```python
from build123d import *

# Parameters (mm, degrees)
EXTRUDE_1_DEPTH         = 13
HOLE_WIZARD_6_2_6_2_1_D = 6.2
HOLE_WIZARD_6_2_6_2_2_D = 6.2
FILLET_1_R              = 3


with BuildPart() as part:
    # 草图1 → 凸台-拉伸1 (new, symmetric)
    with BuildSketch(Plane.XY):
        Polygon((0, 0), (30, 0), (30, 4), (4, 4), (4, 30), (0, 30), align=None)
    extrude(amount=EXTRUDE_1_DEPTH, both=True)

    # Ø6.2 (6.2) 直径孔1 (through all)
    with Locations(Plane(origin=(0, 4, 0), x_dir=(1, 0, 0), z_dir=(0, 1, 0))):
        with Locations((15, 0)):
            Hole(HOLE_WIZARD_6_2_6_2_1_D / 2)

    # Ø6.2 (6.2) 直径孔2 (through all)
    with Locations(Plane(origin=(4, 0, 0), x_dir=(0, 0, -1), z_dir=(1, 0, 0))):
        with Locations((0, 15)):
            Hole(HOLE_WIZARD_6_2_6_2_2_D / 2)

    # 圆角1
    fillet_1_edges = [part.edges().sort_by_distance(p)[0] for p in [
        (4, 30, 0),
        (4, 4, 0),
        (30, 4, 0),
    ]]
    fillet(fillet_1_edges, radius=FILLET_1_R)


solid = part.part
```
Check sheet for the modelled part. Datum: model origin and axes. Units: mm. A direction names the side the tool comes from. Round coordinates to 2 decimals unless told otherwise and drop trailing zeros. Write each loop counter-clockwise with the first axis right and the second up, starting at its lowest first coordinate (ties: lowest second). Pieces come first, ordered by that corner, then holes. Notation, with made-up numbers: (-34.75, 84) -> (0.25, 84) arc R12 ccw to (0.25, 102) -> close; hole circle Ø2 at (68.25, 72). An arc over 180 degrees is marked (long way). One line per question, with ' | ' between items. Start each with the question number.
1. Set-up check for faces 1 (the face through (19, 4, 0)), 2 (the face through (0, 19, 0)): record each of +Z, -Z, +X, -X, +Y, -Y from which the full face is reachable in a straight line by a thin tool's end or side.
2. Sectioned sample at D-D, the plane z = -7. Record the cut outline in (x, y).
3. Scan lines: line 1 along Y through (x, z) = (1.25, 0); line 2 along Z through (x, y) = (15, 1.45); line 3 along X through (y, z) = (20.75, -6.75). Record each from-to range of solid material in increasing order. Write a range as from..to.
4. Sectioned sample at B-B, the plane z = 0. Record the cut outline in (x, y).
5. Depth check by flat-ended pin: pin 1 (4 mm diameter, centred on x = 25, z = 9, fed in from -Y); pin 2 (1 mm diameter, centred on x = 5.5, z = -3, fed in from +Y); pin 3 (3 mm diameter, centred on x = 25, z = -2.5, fed in from +Y); pin 4 (10 mm diameter, centred on y = 7, z = 3.5, fed in from +X). Enter the tip coordinate at first touch or a pass-through.
6. Sectioned sample at A-A, the plane x = 15. Record the cut outline in (y, z).
7. Release check for a two-part mould opening along Z. For faces 3 (the face through (11, 0, 0)), 4 (the face through (3.8, 9.5, 13)), 5 (the face through (17.46, 1.972, 1.886)) record: +Z half, -Z half, draft (parallel to the pull), parting line (faces both ways), or undercut.
Taken from the geometry:
1) face 1: +Z, -Z, +X, +Y | face 2: +Z, -Z, -X, +Y, -Y
2) outline: (0, 0) -> (30, 0) -> (30, 1) arc R3 ccw to (27, 4) -> (7, 4) arc R3 cw to (4, 7) -> (4, 27) arc R3 ccw to (1, 30) -> (0, 30) -> close
3) line 1: y = 0..11.9, 18.1..29.99 | line 2: z = -13..-3.1, 3.1..13 | line 3: x = 0..4
4) outline: (0, 0) -> (11.9, 0) -> (11.9, 4) -> (7, 4) arc R3 cw to (4, 7) -> (4, 11.9) -> (0, 11.9) -> close; (0, 18.1) -> (4, 18.1) -> (4, 27) arc R3 ccw to (1, 30) -> (0, 30) -> close; (18.1, 0) -> (30, 0) -> (30, 1) arc R3 ccw to (27, 4) -> (18.1, 4) -> close
5) pin 1: stops at y = 0 | pin 2: stops at y = 4.76 | pin 3: stops at y = 4 | pin 4: stops at x = 29.83
6) outline: (0, -13) -> (4, -13) -> (4, -3.1) -> (0, -3.1) -> close; (0, 3.1) -> (4, 3.1) -> (4, 13) -> (0, 13) -> close
7) face 3: draft | face 4: +Z half | face 5: undercut
